Read the model definition and answer for the solid it produces. Units are mm, in the model's axes. Face numbers are marked on the shaded views. A direction names the side the tool comes from. Round coordinates to 2 decimals unless told otherwise and drop trailing zeros. Write each loop counter-clockwise with the first axis right and the second up, starting at its lowest first coordinate (ties: lowest second). Pieces come first, ordered by that corner, then holes.
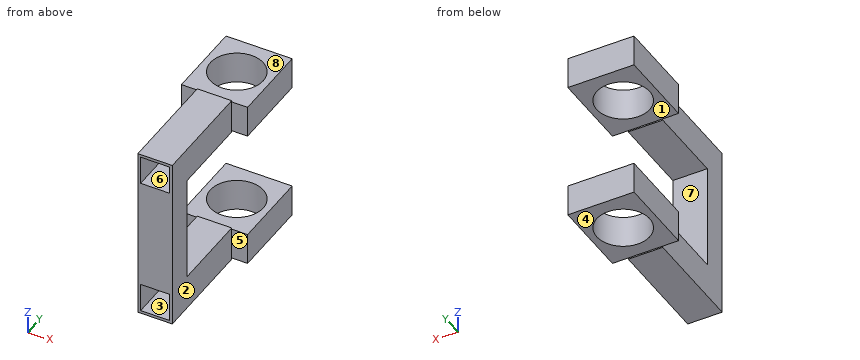
from build123d import *

# Parameters (mm, degrees)
SKETCH1_W                = 13.022
SKETCH1_H                = 40
BOSS_EXTRUDE1_DEPTH      = 10
BOSS_EXTRUDE2_DEPTH      = 30
BOSS_EXTRUDE2_DEPTH_BACK = 10
SKETCH2_W                = 13.022
SKETCH2_H                = 13.022
SKETCH3_W                = 10.902
SKETCH3_H                = 10.902
CUT_EXTRUDE1_DEPTH       = 50
BOSS_EXTRUDE3_START      = 15
SKETCH4_W                = 10.902
SKETCH4_H                = 10.902
BOSS_EXTRUDE3_DEPTH      = 15
SKETCH5_W                = 25
SKETCH5_H                = 12
BOSS_EXTRUDE4_DEPTH      = 30
SKETCH6_R                = 10
CUT_EXTRUDE2_DEPTH       = 100


with BuildPart() as part:
    # Sketch1 → Boss-Extrude1 (new body)
    with BuildSketch(Plane(origin=(0, 0, 0), x_dir=(1, 0, 0), z_dir=(0, 1, 0))):
        with Locations((6.511, 20)):
            Rectangle(SKETCH1_W, SKETCH1_H)
    extrude(amount=BOSS_EXTRUDE1_DEPTH)

    # Sketch2 → Boss-Extrude2 (add, two sides: drawn at the far end of the back side and taken through both)
    with BuildSketch(Plane(origin=(0, 10, 0), x_dir=(1, 0, 0), z_dir=(0, 1, 0)).offset(-BOSS_EXTRUDE2_DEPTH_BACK)):
        with Locations((6.511, 46.511)):
            Rectangle(SKETCH2_W, SKETCH2_H)
        with Locations((6.511, -6.511)):
            Rectangle(SKETCH2_W, SKETCH2_H)
    extrude(amount=BOSS_EXTRUDE2_DEPTH + BOSS_EXTRUDE2_DEPTH_BACK)

    # Sketch3 → Cut-Extrude1 (cut)
    with BuildSketch(Plane(origin=(0, 40, 0), x_dir=(1, 0, 0), z_dir=(0, 1, 0))):
        with Locations((6.511, 46.511)):
            Rectangle(SKETCH3_W, SKETCH3_H)
        with Locations((6.511, -6.511)):
            Rectangle(SKETCH3_W, SKETCH3_H)
    extrude(amount=-CUT_EXTRUDE1_DEPTH, mode=Mode.SUBTRACT)

    # Sketch4 → Boss-Extrude3 (add)
    with BuildSketch(Plane(origin=(0, 10, 0), x_dir=(1, 0, 0), z_dir=(0, 1, 0)).offset(BOSS_EXTRUDE3_START)):
        with Locations((6.511, 46.511)):
            Rectangle(SKETCH4_W, SKETCH4_H)
        with Locations((6.511, -6.511)):
            Rectangle(SKETCH4_W, SKETCH4_H)
    extrude(amount=BOSS_EXTRUDE3_DEPTH)

    # Sketch5 → Boss-Extrude4 (add)
    with BuildSketch(Plane(origin=(0, 40, 0), x_dir=(1, 0, 0), z_dir=(0, 1, 0))):
        with Locations((6.511, 46.511)):
            Rectangle(SKETCH5_W, SKETCH5_H)
        with Locations((6.511, -6.511)):
            Rectangle(SKETCH5_W, SKETCH5_H)
    extrude(amount=BOSS_EXTRUDE4_DEPTH)

    # Sketch6 → Cut-Extrude2 (cut)
    with BuildSketch(Plane.XY.offset(12.511)):
        with Locations((6.511, 55)):
            Circle(SKETCH6_R)
    extrude(amount=-CUT_EXTRUDE2_DEPTH, mode=Mode.SUBTRACT)


solid = part.part
Q1. Section B-B (x = 10.75) is taken. State how many separate pieces and enclosed holes the cut face has, then the cut area to 3 significant figures.
Verdict:
separate pieces: 3
enclosed holes: 0
area: 1,180 mm2
Q2. Section D-D (z = 3.5) is taken. Determine the outline of the cut face in (x, y), then the cut area to 3 significant figures.
Verdict:
outline: (-5.99, 40) - (0, 40) - (0, 0) - (1.06, 0) - (1.06, 25) - (11.96, 25) - (11.96, 0) - (13.02, 0) - (13.02, 40) - (19.01, 40) - (19.01, 70) - (-5.99, 70) - close; hole circle Ø20 at (6.51, 55)
area: 684 mm2
Q3. Determine the mould class of the marked faces 1, 2 and 3 for opening direction X: pulls with the +X half, pulls with the -X half, needs draft (parallel to the pull), parting line crosses it, or undercut.
Verdict:
face 1: needs draft
face 2: pulls with the +X half
face 3: undercut
Q4. Straight lines are drawn through the part: probe 1 along Z at (x, y) = (2.5, 9); probe 2 along Z at (x, y) = (8.5, 13.5); probe 3 along Z at (x, y) = (14.75, 64). For each, find the intervals that lie inside material, in ascending order.
Verdict:
probe 1: z = -53.02 to -51.96, -41.06 to 1.06, 11.96 to 13.02
probe 2: z = -53.02 to -51.96, -41.06 to -40, 0 to 1.06, 11.96 to 13.02
probe 3: z = -52.51 to -40.51, 0.51 to 12.51
Q5. Section A-A (y = 55) is taken. Determine the outline of the cut face in (x, z).
Verdict:
outline: (-5.99, -52.51) - (-3.49, -52.51) - (-3.49, -40.51) - (-5.99, -40.51) - close; (-5.99, 0.51) - (-3.49, 0.51) - (-3.49, 12.51) - (-5.99, 12.51) - close; (16.51, -52.51) - (19.01, -52.51) - (19.01, -40.51) - (16.51, -40.51) - close; (16.51, 0.51) - (19.01, 0.51) - (19.01, 12.51) - (16.51, 12.51) - close
Q6. Which of the six approach directions +Z, -Z, +X, -X, +Y, -Y give full straight-line access (tool end or side, diameter ignored) to the marked faces 4, 5, 6, 7 and 8?
Verdict:
face 4: -Z, +X, -X, +Y
face 5: +Z, -Z, +X, -Y
face 6: -Y
face 7: +X, -X, +Y
face 8: +Z, +X, -X, +Y
Q7. Section C-C (y = 6.5) is taken. Determine the outline of the cut face in (x, z).
Verdict:
outline: (0, -53.02) - (13.02, -53.02) - (13.02, 13.02) - (0, 13.02) - close; hole (1.06, -51.96) - (11.96, -51.96) - (11.96, -41.06) - (1.06, -41.06) - close; hole (1.06, 1.06) - (11.96, 1.06) - (11.96, 11.96) - (1.06, 11.96) - close
Q8. Flat-ended cylindrical pins translate along their axes: pin 1 Ø20 at (y, z) = (19, -15) entering from +X; pin 2 Ø5 at (x, z) = (16, 6.5) entering from -Y; pin 3 Ø12.5 at (x, y) = (7.5, 55) entering from +Z; pin 4 Ø6.5 at (x, z) = (8.5, -18.5) entering from +Y. Find the tip coordinate at first contact, or state that the pin passes through.
Verdict:
pin 1: stops at x = 13.02
pin 2: stops at y = 40
pin 3: passes through
pin 4: stops at y = 10
